Verification items for the finished model (mm, model axes). A direction names the side the tool comes from. Round coordinates to 2 decimals unless told otherwise and drop trailing zeros. Write each loop counter-clockwise with the first axis right and the second up, starting at its lowest first coordinate (ties: lowest second). Pieces come first, ordered by that corner, then holes. Notation, with made-up numbers: (52.5, 18) - (101.5, 18) arc R27 cw to (101.5, 57) - close; hole circle Ø5 at (-17.5, 77). An arc over 180 degrees is marked (long way). Answer as a JSON object with one key per item and string values.
Autodesk Inventor part; units mm, degrees
ref_plane "YZ Plane" through (0, 0, 0) normal (1, 0, 0) x (0, 1, 0)
ref_plane "XZ Plane" through (0, 0, 0) normal (0, 1, 0) x (-1, 0, 0)
ref_plane "XY Plane" through (0, 0, 0) normal (0, 0, 1) x (1, 0, 0)
sketch "Sketch1" plane through (0, 0, 0) normal (0, 0, 1) x (1, 0, 0)
  line L0 (12.7, -25.4) -> (-12.7, -25.4)
  line L1 (-12.7, -25.4) -> (-12.7, 25.4)
  line L2 (-12.7, 25.4) -> (12.7, 25.4)
  line L3 (12.7, 25.4) -> (12.7, -25.4)
  line L4 (12.7, -25.4) -> (-12.7, 25.4) construction
  line L5 (-12.7, -25.4) -> (12.7, 25.4) construction
  line L6 (10.16, 22.86) -> (-10.16, 22.86)
  line L7 (-10.16, 22.86) -> (-10.16, -22.86)
  line L8 (-10.16, -22.86) -> (10.16, -22.86)
  line L9 (10.16, -22.86) -> (10.16, 22.86)
  point P0 (0, 0)
  dimension "d0" = 25.4
  dimension "d1" = 50.8
  dimension "d2" = 2.54
extrude "Extrusion1" add sketch "Sketch1" along normal mid plane 317.5
sketch "Sketch2" plane through (-12.7, 25.4, 158.75) normal (0, 1, 0) x (1, 0, 0)
  point P0 (12.7, 158.75)
  point P1 (12.7, 171.45)
  point P2 (12.7, 146.05)
  dimension "HoleOffset" = 12.7
  dimension "d6" = 12.7
hole "Hole1" at (0, 25.4, -12.7) at (0, 25.4, 12.7) direction (0, -1, 0) diameter 4.1656 end through all
pattern_linear "Rectangular Pattern1" count 31 spacing 50.8 along (0, 0, 1) of "Hole1" first direction both ways yes
properties part number "VersaFrame Side Rail" material "Aluminum 6061"
Q1. Set-up check for faces 5 (the flat face through (0, -22.86, -2)), 6 (the flat face through (-10.4, 2, 158.75)): record each of +Z, -Z, +X, -X, +Y, -Y from which the full face is reachable in a straight line by a thin tool's end or side.
Geometry check:
{"face 5": "+Z, -Z", "face 6": "+Z, +X, -X, +Y, -Y"}
Q2. Section check A-A, the plane x = -6. Record the cut outline in (y, z), then the cut area to 3 significant figures.
Geometry check:
{"outline": "(-25.4, -158.75) - (-22.86, -158.75) - (-22.86, 158.75) - (-25.4, 158.75) - close; (22.86, -158.75) - (25.4, -158.75) - (25.4, 158.75) - (22.86, 158.75) - close", "area": "1,610 mm2"}
Q3. Gauge pin test, flat end, axial feed: P1, Ø2.5, axis at x = 0, z = 139.7, coming from the +Y side. Record the tip position at first contact, or that the pin passes through.
Geometry check:
{"P1": "passes through"}
Q4. Section check C-C, the plane y = 4. Record the cut outline in (x, z), then the cut area to 3 significant figures.
Geometry check:
{"outline": "(-12.7, -158.75) - (-10.16, -158.75) - (-10.16, 158.75) - (-12.7, 158.75) - close; (10.16, -158.75) - (12.7, -158.75) - (12.7, 158.75) - (10.16, 158.75) - close", "area": "1,610 mm2"}
Q5. Material ranges on line 1 along Y through (x, z) = (0.75, -20.5); line 2 along X through (y, z) = (-24, 63); line 3 along X through (y, z) = (11, 34), recorded low to high. Write a range as [from, to].
Geometry check:
{"line 1": "y = [-25.4, -22.86], [22.86, 25.4]", "line 2": "x = [-12.7, -2.02], [2.02, 12.7]", "line 3": "x = [-12.7, -10.16], [10.16, 12.7]"}
Q6. Section check B-B, the plane z = -48. Record the cut outline in (x, y).
Geometry check:
{"outline": "(-12.7, -25.4) - (12.7, -25.4) - (12.7, 25.4) - (-12.7, 25.4) - close; hole (-10.16, -22.86) - (10.16, -22.86) - (10.16, 22.86) - (-10.16, 22.86) - close"}
Q7. Release check for a two-part mould opening along Y. For faces 1 (the flat face through (12.7, 0, -2)), 2 (the flat face through (0, 25.4, -2)), 3 (the flat face through (0, -25.4, -2)), 4 (the flat face through (10.16, 0, -2)) record: released by +Y, released by -Y, zero draft, split by the parting line, or undercut.
Geometry check:
{"face 1": "zero draft", "face 2": "released by +Y", "face 3": "released by -Y", "face 4": "undercut"}
